CAD build for the part. Positions are in the model's coordinates, mm. A direction names the side the tool comes from. Round coordinates to 2 decimals unless told otherwise and drop trailing zeros. Write each loop counter-clockwise with the first axis right and the second up, starting at its lowest first coordinate (ties: lowest second). Pieces come first, ordered by that corner, then holes. Notation, with made-up numbers: (73.25, -30.75) -> (90.25, -30.75) arc R34 cw to (90.25, 8.25) -> close; hole circle Ø3 at (-26, 38.5). An arc over 180 degrees is marked (long way). Put each result on its own line as item: value. Start each with the question number.
1. Flat gauge pins, fed straight in: P1, Ø3, axis at x = 80.5, z = 1, coming from the +Y side; P2, Ø1.5, axis at y = -2.5, z = -1.5, coming from the +X side; P3, Ø4, axis at x = 44, y = 1, coming from the -Z side; P4, Ø1.5, axis at x = 60, y = 0.5, coming from the +Z side. Where does each tip first touch, or does it go through?
2. 3-axis set-ups, long thin cutter, end or side, ignore diameter. For faces 5 (the flat face through (0, 1, 3)), 6 (the conical face through (-3.89, 2.6, 4.49)): which of +Z, -Z, +X, -X, +Y, -Y reach the whole face in a straight line?
3. Drill centre lines: line 1 (X direction, y = -3.5, z = 1); line 2 (X direction, y = -4.75, z = 1.5); line 3 (Y direction, x = 66, z = -0.75). Where is each one in solid material? Low to high. Write a range as from..to.
4. Pull direction Z, two halves, no side cores. Call faces 1 (the flat face through (110, 0, 0)), 2 (the flat face through (-2, 0, 5)), 3 (the cylindrical face through (-0.247, -0.963, -4.334)), 4 (the conical face through (-3.89, 2.58, -4.5)): pulls with the +Z half, pulls with the -Z half, needs draft (parallel to the pull), parting line crosses it, or undercut.
5. Saw through at A-A on x = 91.5. List the corners of the cut face in (y, z), and give its area (3 significant figures).
Autodesk Inventor part; units mm, degrees
ref_plane "Work Plane1" through (1.525, 0, 0) normal (0, 0, 1) x (1, 0, 0)
ref_plane "YZ Plane" through (0, 0, 0) normal (1, 0, 0) x (0, 1, 0)
ref_plane "XZ Plane" through (0, 0, 0) normal (0, 1, 0) x (-1, 0, 0)
sketch "Sketch1" plane through (0, 0, 0) normal (0, 0, 1) x (1, 0, 0)
  line L0 (0, 4.44) -> (0, 3)
  line L1 (92, 3) -> (110, 3)
  line L2 (110, 3) -> (110, 0)
  line L3 (110, 0) -> (-0.5001, 0)
  line L4 (-22.6001, 0) -> (132.1, 0)
  line L5 (-0.5001, 0) -> (-0.5001, 4.44)
  line L6 (-0.5001, 4.44) -> (0, 4.44)
  line L7 (92, 3) -> (91.3864, 3)
  line L8 (91.3864, 3) -> (0, 3)
  line L9 (0, -0.888) -> (0, 5.328)
  dimension "d0" = 110
  dimension "d1" = 18
  dimension "d2" = 6
  dimension "d9" = 0.5001
  dimension "d10" = 8.88
  dimension "d13" = 0.6136
  dimension "d14" = 6
revolve "Body" add sketch "Sketch1" angle 360 about axis through (110, 0, 0) along (-1, 0, 0)
sketch "Sketch2" plane through (-0.5001, 0, 0) normal (-1, 0, 0) x (0, 0, 1)
  line L0 (0, 5.7735) -> (5, 2.8868)
  line L1 (5, 2.8868) -> (5, -2.8868)
  line L2 (5, -2.8868) -> (0, -5.7735)
  line L3 (0, -5.7735) -> (-5, -2.8868)
  line L4 (-5, -2.8868) -> (-5, 2.8868)
  line L5 (-5, 2.8868) -> (0, 5.7735)
  point P0 (0, 0)
  point P1 (0, 0)
  dimension "d11" = 10
extrude "Head" add sketch "Sketch2" along normal blind 3.5
sketch "Sketch4" plane through (0, 0, 0) normal (0, 0, 1) x (1, 0, 0)
  line L0 (-4.0001, 5) -> (-4.0001, 5.7735)
  line L1 (-4.0001, 5.7735) -> (-3.5535, 5.7735)
  line L2 (-3.5535, 5.7735) -> (-4.0001, 5)
  line L3 (-4.7001, 0) -> (0.1999, 0)
  line L4 (-0.5001, 5.7735) -> (-4.0001, 5.7735)
  line L5 (-4.0001, 2.8868) -> (-4.0001, 5.7735)
  dimension "d5" = 30
  dimension "d19" = 10
revolve "Chamfer1" cut sketch "Sketch4" angle 360 about axis through (-10, 0, 0) along (1, 0, 0)
thread "Thread"
chamfer "Chamfer2" distance 0.6135 distance2 0.6136 1 edges at (110, -3, 0) measured on face at (110, 0.3546, -0.935)
ref_plane "Work Plane1" through (1.525, 0, 0) normal (0, 0, 1) x (1, 0, 0)
equation "\"d1\" = GEL"
equation "\"d2\" = GD"
equation "\"d10\" = SD2"
equation "\"d14\" = BDM"
equation "\"d11\" = SW"
equation "\"d3\" = KOH - SD"
equation "\"d5\" = ANG1"
equation "\"d19\" = SW0"
equation "\"d15\" = GEL"
equation "\"d6\" = -0.5 * SPD + 0.5 * GD"
equation "\"GD\" = NND"
equation "\"BDM\" = NND"
equation "\"KOH\" = 4"
equation "\"GEL\" = 18"
equation "\"SW\" = 10"
equation "\"SW0\" = SW"
equation "\"SPD\" = NND - 1.2269 * PTC"
equation "\"SD2\" = 8.88"
equation "\"SD\" = 0.5"
equation "\"ANG1\" = 30deg"
equation "\"GAL\" = 0.61345 * PTC"
equation "\"GUL\" = 0.61345 * PTC"
equation "\"RR\" = 0.25"
equation "\"GD1\" = THREADDIA - 1.2269 * PTC"
equation "\"THREADDIA\" = 6"
equation "\"SDH\" = SD2"
equation "\"TOA\" = 30deg"
equation "\"PTC\" = 1"
equation "\"NND\" = 6"
equation "\"E0\" = 1.155 * SW"
properties part number "ISO 4014 - M6 x 60" material "Stainless Steel, 440C"
Return value:
1. P1: stops at y = 3
1. P2: stops at x = 110
1. P3: stops at z = -3
1. P4: stops at z = 3
2. face 5: +X
2. face 6: +Z, -X, +Y
3. line 1: x = -4..0
3. line 2: x = -4..-0.5
3. line 3: y = -2.9..2.9
4. face 1: needs draft
4. face 2: pulls with the +Z half
4. face 3: parting line crosses it
4. face 4: pulls with the -Z half
5. outline: circle Ø6 at (0, 0)
5. area: 28.3 mm^2
